Geometry: final body of the model. Coordinates: model frame, mm. Face numbers are marked on the shaded views. A direction names the side the tool comes from. Round coordinates to 2 decimals unless told otherwise and drop trailing zeros. Loops run counter-clockwise (first coordinate to the right, second up) from the corner with the lowest first, then second, coordinate; pieces in that order, holes last. Notation, with made-up numbers: M 12,72.5 L 29,72.5 A14 ccw 29,79.5 Z; hole C 28,-8 d3. An arc over 180 degrees is marked long. Answer as a JSON object with one key per item and string values.
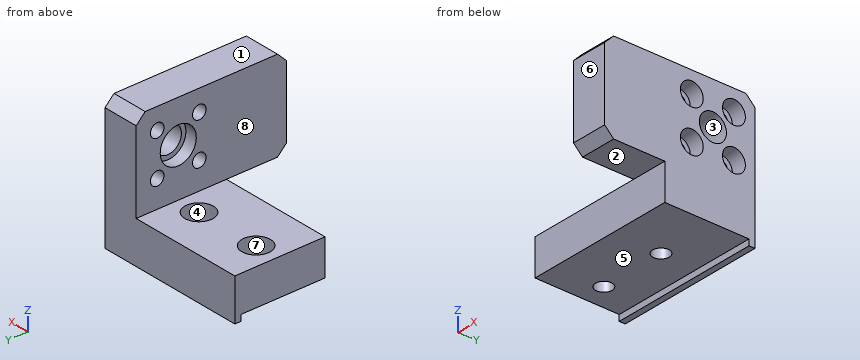
```python
from build123d import *

# Parameters (mm, degrees)
EXTRUDE_1_DEPTH           = 15
SKETCH_2_R                = 6
CUT_EXTRUDE_1_DEPTH       = 4
SKETCH_3_R                = 4.5
CUT_EXTRUDE_2_DEPTH       = 69.271516755
HOLE_WIZARD_1_D           = 4.5
HOLE_WIZARD_1_DEPTH       = 100
HOLE_WIZARD_1_CBORE_D     = 7.6
HOLE_WIZARD_1_CBORE_DEPTH = 5
HOLE_WIZARD_2_D           = 5.5
HOLE_WIZARD_2_DEPTH       = 100
HOLE_WIZARD_2_CBORE_D     = 9.5
HOLE_WIZARD_2_CBORE_DEPTH = 6
SKETCH_8_W                = 12
SKETCH_8_H                = 30
EXTRUDE_2_DEPTH           = 20
CHAMFER_1_SIZE            = 3
SKETCH_10_W               = 2
SKETCH_10_H               = 28
CUT_EXTRUDE_4_DEPTH       = 76.239617224


with BuildPart() as part:
    # 草图1 → 凸台-拉伸1 (new, symmetric)
    with BuildSketch(Plane(origin=(0, 0, 0), x_dir=(1, 0, 0), z_dir=(0, 1, 0))):
        Polygon((-25, 0), (25, 0), (25, -44), (13, -44), (13, -14), (-25, -14), align=None)
    extrude(amount=EXTRUDE_1_DEPTH, both=True)

    # 草图2 → 切除-拉伸1 (cut)
    with BuildSketch(Plane(origin=(13, 0, 0), x_dir=(0, 0, -1), z_dir=(1, 0, 0))):
        with Locations((-30, 1)):
            Circle(SKETCH_2_R)
    extrude(amount=CUT_EXTRUDE_1_DEPTH, mode=Mode.SUBTRACT)

    # 草图3 → 切除-拉伸2 (cut, through all)
    with BuildSketch(Plane(origin=(25, 0, 0), x_dir=(0, 0, -1), z_dir=(1, 0, 0))):
        with Locations((-30, 1)):
            Circle(SKETCH_3_R)
    extrude(amount=-CUT_EXTRUDE_2_DEPTH, mode=Mode.SUBTRACT)

    # 孔1
    with Locations(Plane(origin=(25, 11.754948617, 2.830371217), x_dir=(0, 0, -1), z_dir=(1, 0, 0))):
        with Locations((-20.169628783, -3.754948617), (-34.169628783, -3.754948617), (-20.169628783, -17.754948617), (-34.169628783, -17.754948617)):
            CounterBoreHole(HOLE_WIZARD_1_D / 2, HOLE_WIZARD_1_CBORE_D / 2, HOLE_WIZARD_1_CBORE_DEPTH, depth=HOLE_WIZARD_1_DEPTH)

    # 孔2
    with Locations(Plane(origin=(-5.053295234, -5.294643146, 14), x_dir=(1, 0, 0), z_dir=(0, 0, 1))):
        with Locations((10.053295234, 6.294643146), (-11.946704766, 6.294643146)):
            CounterBoreHole(HOLE_WIZARD_2_D / 2, HOLE_WIZARD_2_CBORE_D / 2, HOLE_WIZARD_2_CBORE_DEPTH, depth=HOLE_WIZARD_2_DEPTH)

    # 草图8 → 凸台-拉伸2 (add)
    with BuildSketch(Plane.XZ.offset(15)):
        with Locations((19, 29)):
            Rectangle(SKETCH_8_W, SKETCH_8_H)
    extrude(amount=EXTRUDE_2_DEPTH)

    # 倒角1
    chamfer_1_edges = [part.edges().sort_by_distance(p)[0] for p in [
        (19, 15, 44),
        (19, -35, 44),
        (19, -35, 14),
    ]]
    chamfer(chamfer_1_edges, length=CHAMFER_1_SIZE)

    # 草图10 → 切除-拉伸4 (cut, through all)
    with BuildSketch(Plane(origin=(25, 0, 0), x_dir=(0, 0, -1), z_dir=(1, 0, 0))):
        with Locations((-1, -1)):
            Rectangle(SKETCH_10_W, SKETCH_10_H)
    extrude(amount=-CUT_EXTRUDE_4_DEPTH, mode=Mode.SUBTRACT)


solid = part.part
```
1) Cut plane C-C on y = 1. Count the separate pieces of the cut face and the enclosed holes in it, and give its area (3 significant figures).
Geometry results:
{"separate pieces": "4", "enclosed holes": "0", "area": "660 mm2"}
2) Cut plane D-D on x = -17. Return the cut outline in (y, z), and give its area (3 significant figures).
Geometry results:
{"outline": "M -15,2 L -1.75,2 L -1.75,8 L -3.75,8 L -3.75,14 L -15,14 Z; M 3.75,2 L 13,2 L 13,0 L 15,0 L 15,14 L 5.75,14 L 5.75,8 L 3.75,8 Z", "area": "274 mm2"}
3) Set-up query: the marked faces 5, 6, 7 and 8. Return all of +Z, -Z, +X, -X, +Y, -Y with unobstructed straight access to the full face (end or side cutting, diameter ignored); none if empty.
Geometry results:
{"face 5": "-Z, +X, -X, -Y", "face 6": "+Z, -Z, +X, -X, -Y", "face 7": "+Z", "face 8": "+Z, -X, +Y, -Y"}
4) Cut plane A-A on y = -6. Return the cut outline in (x, z).
Geometry results:
{"outline": "M -25,2 L 25,2 L 25,19.2 L 20,19.2 L 20,20.75 L 13,20.75 L 13,14 L -25,14 Z; M 13,25.25 L 20,25.25 L 20,26.8 L 25,26.8 L 25,33.2 L 20,33.2 L 20,34.75 L 13,34.75 Z; M 13,39.25 L 20,39.25 L 20,40.8 L 25,40.8 L 25,44 L 13,44 Z"}
5) Pull-direction query (Z, two-part tool) for the marked faces 1, 2, 3 and 4; classes: +Z half, -Z half, draft (parallel to the pull), parting line (faces both ways), or undercut.
Geometry results:
{"face 1": "+Z half", "face 2": "-Z half", "face 3": "undercut", "face 4": "draft"}
6) Cut plane B-B on z = 30. Return the cut outline in (x, y).
Geometry results:
{"outline": "M 13,-35 L 25,-35 L 25,-3.5 L 17,-3.5 L 17,-5 L 13,-5 Z; M 13,7 L 17,7 L 17,5.5 L 25,5.5 L 25,15 L 13,15 Z"}
7) Line query: probe 1 along Y at (x, z) = (23.7, 23); probe 2 along Y at (x, z) = (15.25, 37); probe 3 along X at (y, z) = (-18.5, 27). Output: solid intervals per line, ascending.
Geometry results:
{"probe 1": "-35 to -9.8, -2.2 to 4.2, 11.8 to 15", "probe 2": "-35 to -8.25, -3.75 to 5.75, 10.25 to 15", "probe 3": "13 to 25"}
8) First-contact query: pin 1 (11 mm diameter, centred on x = 5, y = 1, fed in from +Z); pin 2 (1.5 mm diameter, centred on x = -19, z = 15.5, fed in from -Y); pin 3 (5 mm diameter, centred on x = 17.5, y = -14, fed in from -Z); pin 4 (9.5 mm diameter, centred on x = 7.5, z = 9.5, fed in from -Y). Flat tips, straight axial feed; report the tip coordinate or a pass-through.
Geometry results:
{"pin 1": "z = 14", "pin 2": "through", "pin 3": "z = 2", "pin 4": "y = -15"}
